Input: part model. Units: mm. Frame: model coordinates. A direction names the side the tool comes from. Coordinates: 2 decimals unless noted, no trailing zeros. Loops run counter-clockwise (first coordinate to the right, second up) from the corner with the lowest first, then second, coordinate; pieces in that order, holes last.
```python
from build123d import *

# Parameters (mm, degrees)
CROQUIS1_R              = 32
SALIENTE_EXTRUIR1_DEPTH = 5
CROQUIS2_R              = 1.25
CORTAR_EXTRUIR1_DEPTH   = 46.530209751
CORTAR_EXTRUIR2_DEPTH   = 10


with BuildPart() as part:
    # Croquis1 → Saliente-Extruir1 (new body)
    with BuildSketch(Plane.XY):
        Circle(CROQUIS1_R)
    extrude(amount=SALIENTE_EXTRUIR1_DEPTH)

    # Croquis2 → Cortar-Extruir1 (cut, through all)
    with BuildSketch(Plane.XY.offset(5)):
        with Locations((0, 28)):
            Circle(CROQUIS2_R)
        with Locations((19.798989873, 19.798989873)):
            Circle(CROQUIS2_R)
        with Locations((28, 0)):
            Circle(CROQUIS2_R)
        with Locations((19.798989873, -19.798989873)):
            Circle(CROQUIS2_R)
        with Locations((0, -28)):
            Circle(CROQUIS2_R)
        with Locations((-19.798989873, -19.798989873)):
            Circle(CROQUIS2_R)
        with Locations((-28, 0)):
            Circle(CROQUIS2_R)
        with Locations((-19.798989873, 19.798989873)):
            Circle(CROQUIS2_R)
    extrude(amount=-CORTAR_EXTRUIR1_DEPTH, mode=Mode.SUBTRACT)

    # Croquis3 → Cortar-Extruir2 (cut)
    with BuildSketch(Plane.XY.offset(5)):
        with BuildLine():
            Line((-18.875585354, 17.145328155), (-24.086525942, 4.565004714))
            Line((-24.086525942, 4.565004714), (-25.934285007, 5.330371579))
            Line((-25.934285007, 5.330371579), (-26.699651872, 3.482612514))
            Line((-26.699651872, 3.482612514), (-25.332679411, 2.916393981))
            ThreePointArc((-25.332679411, 2.916393981), (-9.758427525, -23.558928079), (19.975111358, -15.850707436))
            Line((19.975111358, -15.850707436), (21.342083819, -16.416925969))
            Line((21.342083819, -16.416925969), (22.107450683, -14.569166904))
            Line((22.107450683, -14.569166904), (20.259691618, -13.803800039))
            Line((20.259691618, -13.803800039), (25.470632207, -1.223476598))
            ThreePointArc((25.470632207, -1.223476598), (9.758427525, 23.558928079), (-18.875585354, 17.145328155))
        make_face()
    extrude(amount=-CORTAR_EXTRUIR2_DEPTH, mode=Mode.SUBTRACT)


solid = part.part
```
Item 1: Section query C-C (y = 22). Output: boundary loops of the cut face in (x, z), then the cut area to 3 significant figures.
Result:
outline: (-23.24, 0) - (-12.89, 0) - (-12.89, 5) - (-23.24, 5) - close; (12.89, 0) - (23.24, 0) - (23.24, 5) - (12.89, 5) - close
area: 103 mm2
Item 2: Mould query, pull axis X, two halves, no side actions, for faces 3 (the face through (-24, 7, 5)), 4 (the face through (-26.026, 3.203, 2.535)). Classes: +X half, -X half, draft (parallel to the pull), parting line (faces both ways), or undercut.
Result:
face 3: draft
face 4: undercut
Item 3: Contact query for flat-ended pins moving along their axis: P1, Ø2, axis at x = -19.8, y = -19.8, coming from the +Z side; P2, Ø1.5, axis at x = 14, z = 1.5, coming from the -Y side; P3, Ø3, axis at x = 12, z = 4.5, coming from the +Y side; P4, Ø3, axis at x = -20, z = 3, coming from the +Y side. Output: stop coordinate, or through.
Result:
P1: passes through
P2: stops at y = -29.13
P3: stops at y = 30.23
P4: stops at y = 26.11
Item 4: Section query A-A (x = 0). Output: boundary loops of the cut face in (y, z), then the cut area to 3 significant figures.
Result:
outline: (-32, 0) - (-29.25, 0) - (-29.25, 5) - (-32, 5) - close; (-26.75, 0) - (-25.5, 0) - (-25.5, 5) - (-26.75, 5) - close; (25.5, 0) - (26.75, 0) - (26.75, 5) - (25.5, 5) - close; (29.25, 0) - (32, 0) - (32, 5) - (29.25, 5) - close
area: 40.0 mm2
Item 5: Reachability of faces 1 (the face through (-21.445, 10.943, 2.535)), 2 (the face through (-24, 7, 0)) from +Z, -Z, +X, -X, +Y, -Y: full face, straight path, thin tool, end or side. Return the list, or none.
Result:
face 1: +Z, -Z
face 2: -Z, +X, -X, +Y, -Y
Item 6: Section query D-D (x = -16). Output: boundary loops of the cut face in (y, z).
Result:
outline: (-27.71, 0) - (-19.86, 0) - (-19.86, 5) - (-27.71, 5) - close; (19.86, 0) - (27.71, 0) - (27.71, 5) - (19.86, 5) - close
Item 7: Line query: L1, parallel to X at y = -9, z = 4.45; L2, parallel to X at y = 12, z = 2.2; L3, parallel to Y at x = 28, z = 3.5. Output: solid intervals per line, ascending.
Result:
L1: x = -30.71 to -23.86, 22.25 to 30.71
L2: x = -29.66 to -21.01, 22.5 to 29.66
L3: y = -15.49 to -1.25, 1.25 to 15.49
